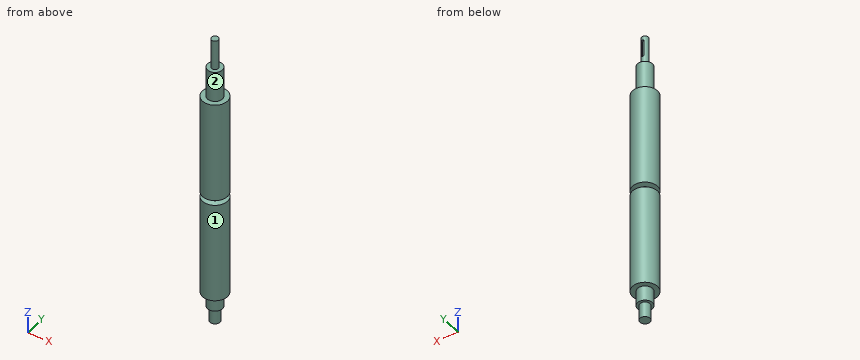
```python
from build123d import *

# Parameters (mm, degrees)
ESQUISSE1_R             = 7
BOSS_EXTRU_1_DEPTH      = 60
ESQUISSE2_R             = 15
BOSS_EXTRU_2_DEPTH      = 61.6
ESQUISSE3_R             = 25
BOSS_EXTRU_3_DEPTH      = 414.8
ESQUISSE4_R             = 15
BOSS_EXTRU_4_DEPTH      = 30
ESQUISSE5_R             = 10
BOSS_EXTRU_5_DEPTH      = 31
ENL_V_MAT_EXTRU_1_DEPTH = 2.96


with BuildPart() as part:
    # Esquisse1 → Boss.-Extru.1 (new body)
    with BuildSketch(Plane.XY):
        Circle(ESQUISSE1_R)
    extrude(amount=BOSS_EXTRU_1_DEPTH)

    # Esquisse2 → Boss.-Extru.2 (add)
    with BuildSketch(Plane(origin=(0, 0, 0), x_dir=(-1, 0, 0), z_dir=(0, 0, -1))):
        Circle(ESQUISSE2_R)
    extrude(amount=BOSS_EXTRU_2_DEPTH)

    # Esquisse3 → Boss.-Extru.3 (add)
    with BuildSketch(Plane(origin=(0, 0, -61.6), x_dir=(-1, 0, 0), z_dir=(0, 0, -1))):
        Circle(ESQUISSE3_R)
    extrude(amount=BOSS_EXTRU_3_DEPTH)

    # Esquisse4 → Boss.-Extru.4 (add)
    with BuildSketch(Plane(origin=(0, 0, -476.4), x_dir=(-1, 0, 0), z_dir=(0, 0, -1))):
        Circle(ESQUISSE4_R)
    extrude(amount=BOSS_EXTRU_4_DEPTH)

    # Esquisse5 → Boss.-Extru.5 (add)
    with BuildSketch(Plane(origin=(0, 0, -506.4), x_dir=(-1, 0, 0), z_dir=(0, 0, -1))):
        Circle(ESQUISSE5_R)
    extrude(amount=BOSS_EXTRU_5_DEPTH)

    # Esquisse7 → Enlèv. mat.-Extru.1 (cut)
    with BuildSketch(Plane(origin=(0, 7, 0), x_dir=(1, 0, 0), z_dir=(0, 1, 0))):
        with BuildLine():
            Line((-2.5, -50), (-2.5, -20))
            ThreePointArc((-2.5, -20), (0, -17.5), (2.5, -20))
            Line((2.5, -20), (2.5, -50))
            ThreePointArc((2.5, -50), (0, -52.5), (-2.5, -50))
        make_face()
    extrude(amount=-ENL_V_MAT_EXTRU_1_DEPTH, mode=Mode.SUBTRACT)

    # Esquisse8 → Enlèvement de matière-Révolution1 (revolve, cut)
    with BuildSketch(Plane(origin=(0, 0, 0), x_dir=(0, 0, -1), z_dir=(1, 0, 0)), mode=Mode.PRIVATE) as enl_vement_de_mati_re_r_volution1_sk:
        Polygon((266, 15.202041029), (264, 25), (274, 25), (272, 15.202041029), align=None)
    revolve(enl_vement_de_mati_re_r_volution1_sk.sketch.rotate(Axis((0, 0, 0), (0, 0, -1)), 90), axis=Axis((0, 0, 0), (0, 0, -1)), mode=Mode.SUBTRACT)  # turned: the seam where the file's is


solid = part.part
```
Could you check a few things on this model? Use its own coordinates, in mm. Face numbers are marked on the shaded views. A direction names the side the tool comes from. Round coordinates to 2 decimals unless told otherwise and drop trailing zeros. Loops run counter-clockwise (first coordinate to the right, second up) from the corner with the lowest first, then second, coordinate; pieces in that order, holes last. Notation, with made-up numbers: (-20, 67.25) - (0, 67.25) arc R8 ccw to (0, 71.25) - close; hole circle Ø7 at (-17.5, 84). An arc over 180 degrees is marked (long way). Answer in a Markdown table with one row per item. Add a question column.
(1) I'm going to push flat-ended pins straight in: pin 1 (0.7 mm diameter, centred on y = 5.5, z = 28, fed in from -X); pin 2 (2 mm diameter, centred on y = 11.5, z = -297, fed in from +X); pin 3 (8 mm diameter, centred on y = 10.5, z = -316.5, fed in from +X). Where does each tip first touch, or does it pass through?
(2) If we section it at A-A (z = -355): Please give me the cut outline in (x, y), plus the area to 3 significant figures.
(3) I need wall thicknesses on line 1 along Z through (x, y) = (-21, -8); line 2 along Z through (x, y) = (-10.5, -21.5); line 3 along Z through (x, y) = (13.5, -3.5). Which ranges of each line are inside material? Lowest first, please.
(4) For the marked faces 1 and 2, which set-ups out of +Z, -Z, +X, -X, +Y, -Y let a thin tool reach every point of the face, with its end or its side?
Model answer:
| question | item | result |
|---|---|---|
| 1 | pin 1 | stops at x = -4.74 |
| 1 | pin 2 | stops at x = 22.69 |
| 1 | pin 3 | stops at x = 24.14 |
| 2 | outline | circle Ø50 at (0, 0) |
| 2 | area | 1,960 mm² |
| 3 | line 1 | z = -476.4 to -273.48, -264.52 to -61.6 |
| 3 | line 2 | z = -476.4 to -273.78, -264.22 to -61.6 |
| 3 | line 3 | z = -506.4 to 0 |
| 4 | face 1 | +Z, -Z |
| 4 | face 2 | +Z |
